Design review of the part built by this model. Coordinates are the model's own, in mm. A direction names the side the tool comes from. Coordinates: 2 decimals unless noted, no trailing zeros. Write each loop counter-clockwise with the first axis right and the second up, starting at its lowest first coordinate (ties: lowest second). Pieces come first, ordered by that corner, then holes. Notation, with made-up numbers: (29, 16.5) - (64, 16.5) arc R21 cw to (64, 33.5) - close; hole circle Ø6 at (50, 69). An arc over 180 degrees is marked (long way). Answer as a JSON object with one key per item and string values.
Autodesk Inventor part; units mm, degrees
ref_plane "YZ Plane" through (0, 0, 0) normal (1, 0, 0) x (0, 1, 0)
ref_plane "XZ Plane" through (0, 0, 0) normal (0, 1, 0) x (-1, 0, 0)
ref_plane "XY Plane" through (0, 0, 0) normal (0, 0, 1) x (1, 0, 0)
sketch "Sketch1" plane through (0, 0, 0) normal (0, 0, 1) x (1, 0, 0)
  line L0 (-105.918, -44.45) -> (105.918, -44.45)
  line L1 (105.918, -44.45) -> (105.918, 44.45)
  line L2 (105.918, 44.45) -> (-105.918, 44.45)
  line L3 (-105.918, 44.45) -> (-105.918, -44.45)
  line L4 (-29.718, 44.45) -> (-29.718, -44.45) construction
  line L5 (29.718, 44.45) -> (29.718, -44.45) construction
  line L6 (-105.918, 19.05) -> (105.918, 19.05) construction
  line L7 (-105.918, -19.05) -> (105.918, -19.05) construction
  line L8 (-67.818, 44.45) -> (-67.818, -44.45) construction
  line L9 (67.818, 44.45) -> (67.818, -44.45) construction
  line L10 (-105.918, 12.446) -> (-29.718, 12.446)
  line L11 (-29.718, 12.446) -> (-29.718, 25.654)
  line L12 (-29.718, 25.654) -> (-105.918, 25.654)
  line L13 (-105.918, 25.654) -> (-105.918, 12.446)
  line L14 (-105.918, 12.446) -> (-29.718, 25.654) construction
  line L15 (-29.718, 12.446) -> (-105.918, 25.654) construction
  line L16 (29.718, -25.654) -> (105.918, -25.654)
  line L17 (105.918, -25.654) -> (105.918, -12.446)
  line L18 (105.918, -12.446) -> (29.718, -12.446)
  line L19 (29.718, -12.446) -> (29.718, -25.654)
  line L20 (29.718, -25.654) -> (105.918, -12.446) construction
  line L21 (105.918, -25.654) -> (29.718, -12.446) construction
  point P0 (0, 0)
  point P1 (-67.818, 19.05)
  point P2 (67.818, -19.05)
  dimension "d2" = 29.718
  dimension "d3" = 29.718
  dimension "d4" = 19.05
  dimension "d5" = 19.05
  dimension "d6" = 67.818
  dimension "d7" = 67.818
  dimension "d9" = 13.208
  dimension "d10" = 76.2
  dimension "d11" = 105.918
  dimension "d12" = 44.45
  dimension "d15" = 105.918
  dimension "d16" = 44.45
extrude "Extrusion1" add sketch "Sketch1" against normal blind 5.842 contours L3 L10 L11 L12 L2 L1 L18 L19 L16 L0
sketch "Sketch2" plane through (0, 0, 0) normal (0, 0, 1) x (1, 0, 0)
  point P0 (0, 0)
  point P1 (0, 31.75)
  point P2 (0, 6.35)
  point P3 (0, -6.35)
  point P4 (0, -31.75)
  dimension "d17" = 25.4
  dimension "d18" = 6.35
  dimension "d19" = 6.35
  dimension "d20" = 25.4
hole "Hole1" at (0, 31.75, 0) at (0, 6.35, 0) at (0, -6.35, 0) at (0, -31.75, 0) direction (0, 0, -1) diameter 5.1054 end through all
sketch "Sketch4" plane through (0, 0, 0) normal (0, 0, 1) x (1, 0, 0)
  line L0 (-105.918, -44.45) -> (-105.918, 12.446) construction
  line L1 (-105.918, -19.05) -> (0, -19.05) construction
  circle A0 centre (-86.868, -19.05) radius 9.525
  circle A1 centre (-61.468, -19.05) radius 9.525
  circle A2 centre (-36.068, -19.05) radius 9.525
  line L2 (0, 19.05) -> (105.8361, 19.05) construction
  circle A3 centre (86.868, 19.05) radius 9.525
  line L3 (105.918, -12.446) -> (105.918, 44.45)
  circle A4 centre (61.468, 19.05) radius 9.525
  circle A5 centre (36.068, 19.05) radius 9.525
  point P0 (0, 0)
  dimension "d28" = 19.05
  dimension "d29" = 19.05
  dimension "d32" = 25.4
  dimension "d37" = 19.05
  dimension "d38" = 19.05
  dimension "d39" = 19.05
  dimension "d40" = 19.05
  dimension "d43" = 25.4
extrude "Extrusion2" cut sketch "Sketch4" against normal through all
equation "\"d9\" = slotWidth"
equation "\"d10\" = slotLength"
equation "\"d13\" = plateThickness"
equation "\"plateWidth\" = 2 * offsetForBracketHoles + 2 * slotLength + 2 * edgeForSlot"
equation "\"plateHeight\" = 88.9"
equation "\"offsetForBracketHoles\" = 29.718"
equation "\"slotLength\" = 76.2"
equation "\"verticalCenterLineOfSlot\" = 19.05"
equation "\"cylinderDiameter\" = 12.7"
equation "\"centerLineOfBracket\" = 17.526"
equation "\"horizontalCenterLineOfSlot\" = 0.5 * slotLength + offsetForBracketHoles"
equation "\"plateThickness\" = 5.842"
equation "\"edgeForSlot\" = 0"
equation "\"centerLineMiddleBracket\" = 14.224"
equation "\"boltCentersForBracket\" = 25.4"
equation "\"printerOffset\" = 0.508"
properties part number "vexPlate" material "PET Plastic"
(1) The part is to be moulded in two halves that separate along X. For faces 1 (the face through (95.667, 15.402, -2.88)), 2 (the face through (-29.718, 19, -3)), 3 (the face through (-1, 1, -5.842)), 4 (the face through (29.718, -19, -3)), say which applies: pulls with the +X half, pulls with the -X half, needs draft (parallel to the pull), parting line crosses it, or undercut.
Solved:
{"face 1": "undercut", "face 2": "pulls with the -X half", "face 3": "needs draft", "face 4": "pulls with the +X half"}
(2) Take a section at C-C, the plane z = -4.4. Give the number of separate pieces and of enclosed holes in the cut face, and give its area (3 significant figures).
Solved:
{"separate pieces": "1", "enclosed holes": "10", "area": "15,000 mm^2"}
(3) For pin 1 (11.5 mm diameter, centred on x = -36.068, y = -19.05, fed in from -Z); pin 2 (1.8 mm diameter, centred on y = 18.5, z = -4, fed in from -X), all flat-tipped, find the tip position at first contact; note any pin that passes through.
Solved:
{"pin 1": "passes through", "pin 2": "stops at x = -29.72"}
(4) To check wall thickness, follow line 1 (Y direction, x = 0, z = -3.8); line 2 (X direction, y = -19, z = -5.1); line 3 (X direction, y = 18.5, z = -3.3). State the ranges of each line that lie inside material, in increasing order. Write a range as from..to.
Solved:
{"line 1": "y = -44.45..-34.3, -29.2..-8.9, -3.8..3.8, 8.9..29.2, 34.3..44.45", "line 2": "x = -105.92..-96.39, -77.34..-70.99, -51.94..-45.59, -26.54..29.72", "line 3": "x = -29.72..26.56, 45.58..51.96, 70.98..77.36, 96.38..105.92"}
(5) Take a section at D-D, the plane x = -61.5. Write out the cut boundary in (y, z).
Solved:
{"outline": "(-44.45, -5.84) - (-28.57, -5.84) - (-28.57, 0) - (-44.45, 0) - close; (-9.53, -5.84) - (12.45, -5.84) - (12.45, 0) - (-9.53, 0) - close; (25.65, -5.84) - (44.45, -5.84) - (44.45, 0) - (25.65, 0) - close"}
(6) Take a section at A-A, the plane y = 6.35. Write out the cut boundary in (x, z), and give its area (3 significant figures).
Solved:
{"outline": "(-105.92, -5.84) - (-2.55, -5.84) - (-2.55, 0) - (-105.92, 0) - close; (2.55, -5.84) - (105.92, -5.84) - (105.92, 0) - (2.55, 0) - close", "area": "1,210 mm^2"}
(7) Take a section at B-B, the plane x = 0. Write out the cut boundary in (y, z).
Solved:
{"outline": "(-44.45, -5.84) - (-34.3, -5.84) - (-34.3, 0) - (-44.45, 0) - close; (-29.2, -5.84) - (-8.9, -5.84) - (-8.9, 0) - (-29.2, 0) - close; (-3.8, -5.84) - (3.8, -5.84) - (3.8, 0) - (-3.8, 0) - close; (8.9, -5.84) - (29.2, -5.84) - (29.2, 0) - (8.9, 0) - close; (34.3, -5.84) - (44.45, -5.84) - (44.45, 0) - (34.3, 0) - close"}
(8) Tool access review of faces 5 (the face through (-67, 25.654, -3)), 6 (the face through (105.918, 16, -3)), 7 (the face through (68, -12.446, -3)): name each direction out of +Z, -Z, +X, -X, +Y, -Y from which nothing blocks a thin tool from reaching the whole face with its end or side.
Solved:
{"face 5": "+Z, -Z, -X", "face 6": "+Z, -Z, +X, +Y, -Y", "face 7": "+Z, -Z, +X"}
